Check sheet for the modelled part. Datum: model origin and axes. Units: mm. Coordinates: 2 decimals unless noted, no trailing zeros. Loops run counter-clockwise (first coordinate to the right, second up) from the corner with the lowest first, then second, coordinate; pieces in that order, holes last. Notation, with made-up numbers: M -3,78.25 L 50,78.25 A14 ccw 50,101.25 Z; hole C 62.25,55.25 d2. An arc over 180 degrees is marked long. Answer in a Markdown table with one row per item. Add a question column.
```python
from build123d import *

# Parameters (mm, degrees)
SKETCH1_W           = 40
SKETCH1_H           = 17
BOSS_EXTRUDE1_DEPTH = 22
SKETCH2_R           = 1.5
CUT_EXTRUDE1_DEPTH  = 22
SKETCH3_R           = 1.5
CUT_EXTRUDE2_DEPTH  = 22


with BuildPart() as part:
    # Sketch1 → Boss-Extrude1 (new body)
    with BuildSketch(Plane(origin=(0, 0, 0), x_dir=(1, 0, 0), z_dir=(0, 1, 0))):
        Rectangle(SKETCH1_W, SKETCH1_H)
    extrude(amount=BOSS_EXTRUDE1_DEPTH)

    # Sketch2 → Cut-Extrude1 (cut)
    with BuildSketch(Plane(origin=(0, 22, 0), x_dir=(1, 0, 0), z_dir=(0, 1, 0))):
        with Locations(Location((-17, -5.5, 0), (0, 0, 270))):
            Circle(SKETCH2_R)
    extrude(amount=-CUT_EXTRUDE1_DEPTH, mode=Mode.SUBTRACT)

    # Sketch3 → Cut-Extrude2 (cut)
    with BuildSketch(Plane(origin=(0, 22, 0), x_dir=(1, 0, 0), z_dir=(0, 1, 0))):
        with Locations(Location((1.5, -5.5, 0), (0, 0, 270))):
            Circle(SKETCH3_R)
    extrude(amount=-CUT_EXTRUDE2_DEPTH, mode=Mode.SUBTRACT)


solid = part.part
```
Q1. Thickness scan on L1, parallel to X at y = 20.25, z = 5.5; L2, parallel to X at y = 16.5, z = 4.5. Record the ranges inside material, lowest first.
Q2. Cross-section at A-A (x = -17). Record the cut outline in (y, z), plus the area to 3 significant figures.
Q3. Cross-section at B-B (z = 5.5). Record the cut outline in (x, y), plus the area to 3 significant figures.
Q4. Cross-section at C-C (y = 8.5). Record the cut outline in (x, z).
Q5. Go/stop test with a flat-tipped pin: pin 1 (2 mm diameter, centred on x = 5.5, z = -1.5, fed in from -Y). Record where the tip stops, or that it passes through.
Q6. Mould release check, pull along X, two halves, no side actions. Record for faces 1 (the face through (20, 11, 0)), 2 (the face through (-15.513, 11.154, 5.305)), 3 (the face through (2.51, 11.15, 4.39)), 4 (the face through (0, 0, 0)): released by +X, released by -X, zero draft, split by the parting line, or undercut.
Answer key:
| question | item | result |
|---|---|---|
| 1 | L1 | -20 to -18.5, -15.5 to 0, 3 to 20 |
| 1 | L2 | -20 to -18.12, -15.88 to 0.38, 2.62 to 20 |
| 2 | outline | M 0,-8.5 L 22,-8.5 L 22,4 L 0,4 Z; M 0,7 L 22,7 L 22,8.5 L 0,8.5 Z |
| 2 | area | 308 mm^2 |
| 3 | outline | M -20,0 L -18.5,0 L -18.5,22 L -20,22 Z; M -15.5,0 L 0,0 L 0,22 L -15.5,22 Z; M 3,0 L 20,0 L 20,22 L 3,22 Z |
| 3 | area | 748 mm^2 |
| 4 | outline | M -20,-8.5 L 20,-8.5 L 20,8.5 L -20,8.5 Z; hole C -17,5.5 d3; hole C 1.5,5.5 d3 |
| 5 | pin 1 | y = 0 |
| 6 | face 1 | released by +X |
| 6 | face 2 | undercut |
| 6 | face 3 | undercut |
| 6 | face 4 | zero draft |
